```python
from build123d import *

# Parameters (mm, degrees)
SKETCH2_R           = 5.461
BOSS_EXTRUDE1_DEPTH = 12.7
FILLET1_R           = 3.81


with BuildPart() as part:
    # Sketch1 → Revolve1 (revolve)
    with BuildSketch(Plane.XY, mode=Mode.PRIVATE) as revolve1_sk:
        Polygon((0, 0), (0, 38.1), (3.81, 38.1), (5.461, 0), align=None)
    revolve(revolve1_sk.sketch.rotate(Axis((0, 0, 0), (0, 1, 0)), 90), axis=Axis((0, 0, 0), (0, 1, 0)))

    # Sketch2 → Boss-Extrude1 (add)
    with BuildSketch(Plane(origin=(0, 0, 0), x_dir=(-1, 0, 0), z_dir=(0, -1, 0))):
        with Locations(Location((0, 0, 0), (0, 0, 90))):
            Circle(SKETCH2_R)
    extrude(amount=BOSS_EXTRUDE1_DEPTH)

    # Fillet1
    fillet1_edges = [part.edges().sort_by_distance(p)[0] for p in [
        (0, 38.1, 3.81),
    ]]
    fillet(fillet1_edges, radius=FILLET1_R)


solid = part.part
```
Geometry check sheet. Reference: the model listing, model coordinates, mm. Coordinates: 2 decimals unless noted, no trailing zeros. Loops run counter-clockwise (first coordinate to the right, second up) from the corner with the lowest first, then second, coordinate; pieces in that order, holes last.
Item 1: Go/stop test with flat-tipped pins: pin 1 Ø1 at (x, y) = (1.5, 2.5) entering from +Z; pin 2 Ø1.5 at (x, z) = (-4, 1.5) entering from +Y; pin 3 Ø1.5 at (y, z) = (31.5, 1) entering from +X. Record where each tip stops, or that it passes through.
Item 2: Thickness scan on line 1 (Y direction, x = -3, z = 0.5); line 2 (X direction, y = -2, z = 3.25); line 3 (Z direction, x = -0.25, y = 11). Record the ranges inside material, lowest first.
Item 3: Sectioned sample at B-B, the plane y = 16.5. Record the boundary of the cut face in (x, z), then the cut area to 3 significant figures.
Item 4: Sectioned sample at A-A, the plane y = 6. Record the boundary of the cut face in (x, z), then the cut area to 3 significant figures.
Check result:
1. pin 1: stops at z = 5.26
1. pin 2: stops at y = 36.09
1. pin 3: stops at x = 4.1
2. line 1: y = -12.7 to 36.78
2. line 2: x = -4.39 to 4.39
2. line 3: z = -4.98 to 4.98
3. outline: circle Ø9.49 at (0, 0)
3. area: 70.8 mm2
4. outline: circle Ø10.4 at (0, 0)
4. area: 85.0 mm2
